from build123d import *

# Parameters (mm, degrees)
SKETCH_1_R      = 3
EXTRUDE_1_DEPTH = 10
SKETCH_2_R      = 1.5
EXTRUDE_2_DEPTH = 6
M3X0_5_1_D      = 2.5
M3X0_5_1_DEPTH  = 8.5
M3X0_5_1_TIP    = 0.751075774
CHAMFER_1_SIZE  = 0.4


with BuildPart() as part:
    # ｽｹｯﾁ1 → ﾎﾞｽ - 押し出し1 (new body)
    with BuildSketch(Plane(origin=(0, 0, 0), x_dir=(0, 1, 0), z_dir=(0, 0, 1))):
        Circle(SKETCH_1_R)
    extrude(amount=EXTRUDE_1_DEPTH)

    # ｽｹｯﾁ2 → ﾎﾞｽ - 押し出し2 (add)
    with BuildSketch(Plane.XY.offset(10)):
        Circle(SKETCH_2_R)
    extrude(amount=EXTRUDE_2_DEPTH)

    # M3x0.5 ねじ穴1
    with Locations(Plane(origin=(0, 0, 0), x_dir=(1, 0, 0), z_dir=(0, 0, -1))):
        with Locations((0, 0)):
            Hole(M3X0_5_1_D / 2, depth=M3X0_5_1_DEPTH)
            with Locations((0, 0, -(M3X0_5_1_DEPTH + M3X0_5_1_TIP / 2))):  # 118° drill point
                Cone(0, M3X0_5_1_D / 2, M3X0_5_1_TIP, mode=Mode.SUBTRACT)

    # 面取り1
    chamfer_1_edges = [part.edges().sort_by_distance(p)[0] for p in [
        (1.25, 0, 0),
        (-1.5, 0, 16),
    ]]
    chamfer(chamfer_1_edges, length=CHAMFER_1_SIZE)


solid = part.part
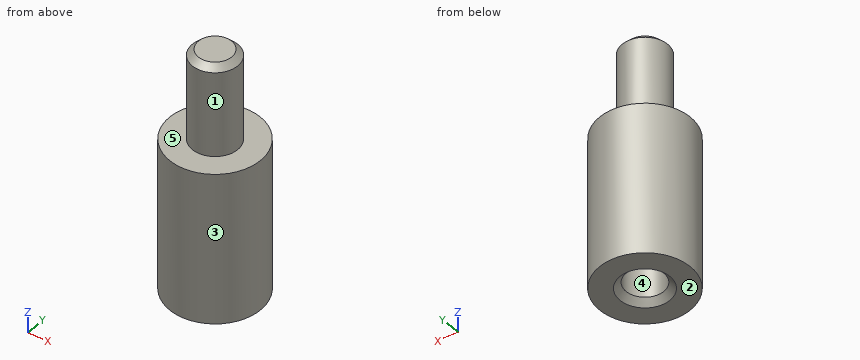
Input: part model. Units: mm. Frame: model coordinates. Face numbers are marked on the shaded views. A direction names the side the tool comes from. Round coordinates to 2 decimals unless told otherwise and drop trailing zeros. Loops run counter-clockwise (first coordinate to the right, second up) from the corner with the lowest first, then second, coordinate; pieces in that order, holes last. Notation, with made-up numbers: (5.25, -3) -> (16.25, -3) arc R21 cw to (16.25, 7) -> close; hole circle Ø6 at (64.25, -16). An arc over 180 degrees is marked (long way). Answer as a JSON object with one key per item and string values. Group by question number.
1) Section query D-D on y = -2.35. Output: boundary loops of the cut face in (x, z).
2) Section query A-A on z = 13. Output: boundary loops of the cut face in (x, y).
3) Ray query, L1, parallel to Y at x = 0, z = 7; L2, parallel to Z at x = -0.65, y = -1.75. Return the intervals inside material, ascending.
4) Draft query along X for the marked faces 3, 4 and 5. Return one class per face: +X half, -X half, draft (parallel to the pull), parting line (faces both ways), or undercut.
5) Section query B-B on z = 4. Output: boundary loops of the cut face in (x, y).
6) Pin query (flat end, axial travel): pin 1 (3 mm diameter, centred on x = -0.5, z = 14, fed in from -Y); pin 2 (3 mm diameter, centred on x = 0, y = 0, fed in from -Z). Return the tip coordinate at first contact, or that it passes through.
7) Section query C-C on x = -2.5. Output: boundary loops of the cut face in (y, z), plus the area to 3 significant figures.
8) Reachability of the marked faces 1 and 2 from +Z, -Z, +X, -X, +Y, -Y: full face, straight path, thin tool, end or side. Return the list, or none.
Reply:
{
 "1": {"outline": "(-1.86, 0) -> (1.86, 0) -> (1.86, 10) -> (-1.86, 10) -> close"},
 "2": {"outline": "circle Ø3 at (0, 0)"},
 "3": {"L1": "y = -3 to -1.25, 1.25 to 3", "L2": "z = 0 to 10"},
 "4": {"face 3": "parting line", "face 4": "undercut", "face 5": "draft"},
 "5": {"outline": "circle Ø6 at (0, 0); hole circle Ø2.5 at (0, 0)"},
 "6": {"pin 1": "stops at y = -1.5", "pin 2": "stops at z = 0.15"},
 "7": {"outline": "(-1.66, 0) -> (1.66, 0) -> (1.66, 10) -> (-1.66, 10) -> close", "area": "33.2 mm2"},
 "8": {"face 1": "+Z", "face 2": "-Z, +X, -X, +Y, -Y"}
}
